Model file for the job. Use its own axes, mm. A direction names the side the tool comes from. Give positions to 0.01 mm unless a question says otherwise; leave off trailing zeros. Loops run counter-clockwise (first coordinate to the right, second up) from the corner with the lowest first, then second, coordinate; pieces in that order, holes last. Notation, with made-up numbers: M 84,-19.5 L 124,-19.5 A31 ccw 124,11.5 Z; hole C 38,69 d8. An arc over 180 degrees is marked long. Use CSV: the item, a comma, the result in double quotes. Start each with the question number.
(1) Slice it at D-D on y = 2.25. List the corners of the cut face in (x, z), and give its area (3 significant figures).
(2) Slice it at A-A on x = 0. List the corners of the cut face in (y, z), and give its area (4 significant figures).
(3) Slice it at C-C on z = 3.25. List the corners of the cut face in (x, y), and give its area (3 significant figures).
(4) Wall check: line 1 along Z through (x, y) = (-5, 3); line 2 along X through (y, z) = (0.25, 12.5); line 3 along Y through (x, z) = (0, 16). Give the ranges that are in metal, low to high. Write a range as from..to.
(5) Flat gauge pins, fed straight in: P1, Ø12, axis at y = 0, z = 3, coming from the +X side; P2, Ø3, axis at y = -4, z = 14.5, coming from the +X side; P3, Ø12, axis at x = -7, z = 15, coming from the +Y side; P4, Ø2.5, axis at x = 3.5, y = -0.5, coming from the +Z side. Where does each tip first touch, or does it go through?
(6) Tool access for faces 4 (the face through (-1.08, -4.88, 10.05)), 5 (the face through (0, -1.5, 20)), 6 (the face through (0, -5, 21.7)): list every direction of +Z, -Z, +X, -X, +Y, -Y with a clear straight run to the whole face (end or side of a thin tool).
(7) Two-plate mould, pull along Y, no slides. Class faces 1 (the face through (-5, -2, 13.7)), 2 (the face through (-0.867, -3.905, 3.204)), 3 (the face through (0, 0, 18.2)): pulls with the +Y half, pulls with the -Y half, needs draft (parallel to the pull), parting line crosses it, or undercut.
(8) Slice it at B-B on y = 0. List the corners of the cut face in (x, z), and give its area (3 significant figures).
```python
from build123d import *

# Parameters (mm, degrees)
F0_R     = 4
F1_DEPTH = 6.5
F2_R     = 5
F3_DEPTH = 7.2
F4_R     = 10
F5_DEPTH = 4.5
F7_DEPTH = 3.5


with BuildPart() as f1:
    # F0 (on Top) → F1 (new body)
    with BuildSketch(Plane.XY):
        Circle(F0_R)
    extrude(amount=F1_DEPTH)

    # F2 (on face) → F3 (join)
    with BuildSketch(Plane.XY.offset(6.5)):
        Circle(F2_R)
    extrude(amount=F3_DEPTH)

    # F4 (on face) → F5 (join)
    with BuildSketch(Plane.XY.offset(13.7)):
        Circle(F4_R)
    extrude(amount=F5_DEPTH)

    # F6 (on face) → F7 (join)
    with BuildSketch(Plane.XY.offset(18.2)):
        with BuildLine():
            ThreePointArc((-9.8868599666, -1.5), (0, -10), (9.8868599666, -1.5))
            Line((9.8868599666, -1.5), (-9.8868599666, -1.5))
        make_face()
        with BuildLine():
            Line((-9.8868599666, 1.5), (9.8868599666, 1.5))
            ThreePointArc((9.8868599666, 1.5), (0, 10), (-9.8868599666, 1.5))
        make_face()
    extrude(amount=F7_DEPTH)


solid = f1.part
```
Reply:
1,outline,"M -9.74,13.7 L -4.47,13.7 L -4.47,6.5 L -3.31,6.5 L -3.31,0 L 3.31,0 L 3.31,6.5 L 4.47,6.5 L 4.47,13.7 L 9.74,13.7 L 9.74,21.7 L -9.74,21.7 Z"
1,area,"263 mm^2"
2,outline,"M -10,13.7 L -5,13.7 L -5,6.5 L -4,6.5 L -4,0 L 4,0 L 4,6.5 L 5,6.5 L 5,13.7 L 10,13.7 L 10,21.7 L 1.5,21.7 L 1.5,18.2 L -1.5,18.2 L -1.5,21.7 L -10,21.7 Z"
2,area,"273.5 mm^2"
3,outline,"C 0,0 d8"
3,area,"50.3 mm^2"
4,line 1,"z = 13.7..21.7"
4,line 2,"x = -4.99..4.99"
4,line 3,"y = -10..10"
5,P1,"stops at x = 5"
5,P2,"stops at x = 9.68"
5,P3,"stops at y = 9.95"
5,P4,"stops at z = 21.7"
6,face 4,"-Z"
6,face 5,"+Z, +X, -X"
6,face 6,"+Z, +X, -X, +Y, -Y"
7,face 1,"needs draft"
7,face 2,"parting line crosses it"
7,face 3,"undercut"
8,outline,"M -10,13.7 L -5,13.7 L -5,6.5 L -4,6.5 L -4,0 L 4,0 L 4,6.5 L 5,6.5 L 5,13.7 L 10,13.7 L 10,18.2 L -10,18.2 Z"
8,area,"214 mm^2"
